Geometry check sheet. Reference: the model listing, model coordinates, mm. Round coordinates to 2 decimals unless told otherwise and drop trailing zeros. Order: outer loops, then holes, each group sorted by start corner. A loop starts at its lowest first (then second) coordinate and runs counter-clockwise, first axis right, second up. Notation, with made-up numbers: (60, 7.5) - (75, 7.5) arc R13 cw to (75, 23.5) - close; hole circle Ø5 at (-2.75, 37.25). An arc over 180 degrees is marked (long way). Return JSON: item names as keys, results as strings. Group by question number.
Q1. Material ranges on line 1 along Z through (x, y) = (-6, 3); line 2 along Y through (x, z) = (0, 8.75) (3 decimals); line 3 along X through (y, z) = (1, 5), recorded low to high.
Q2. Sectioned sample at A-A, the plane x = 0. Record the cut outline in (y, z) (3 decimals), then the cut area to 3 significant figures.
Q3. Gauge pin test, flat ends, axial feed: pin 1 Ø6 at (x, z) = (-8.5, 1) entering from +Y; pin 2 Ø5 at (x, z) = (-9.5, 4.5) entering from +Y; pin 3 Ø5 at (x, y) = (0, 0) entering from -Z; pin 4 Ø2 at (y, z) = (1, 2) entering from +X. Record the tip position at first contact, or that the pin passes through.
Q4. Draft check along Y on faces 1 (the cylindrical face through (-11.34, -0.65, 6.15)), 2 (the flat face through (-9.713, -0.012, -0.176)), 3 (the conical face through (9.553, 3.008, 5.127)), 4 (the cylindrical face through (-3.15, -2.41, 6.57)). Enter one of: pulls with the +Y half, pulls with the -Y half, needs draft (parallel to the pull), parting line crosses it, or undercut.
```python
from build123d import *

# Parameters (mm, degrees)
F0_R     = 8.895
F2_R     = 11.725
F4_R     = 3.965
F5_DEPTH = 12.95
F9_DEPTH = 13.225


with BuildPart() as f3:
    # F0 (on Top) → F3 section 0
    with BuildSketch(Plane.XY):
        Circle(F0_R)
    # F2 (on offset) → F3 section 1
    with BuildSketch(Plane.XY.offset(12.95)):
        Circle(F2_R)
    loft()

    # F4 (on face) → F5 (cut)
    with BuildSketch(Plane.XY.offset(12.95)):
        Circle(F4_R)
    extrude(amount=-F5_DEPTH, mode=Mode.SUBTRACT)

    # F8 (on face) → F9 (join)
    with BuildSketch(Plane(origin=(-0.370918, 0, 1.775485), x_dir=(0.978867, 0, 0.204496), z_dir=(0.204496, 0, -0.978867))):
        with BuildLine():
            ThreePointArc((-8.665283, 0.869945), (-9.857422, 0.644661), (-10.88518, -5.5e-05))
            ThreePointArc((-10.88518, -5.5e-05), (-9.857417, -0.644773), (-8.665273, -0.870055))
            ThreePointArc((-8.665273, -0.870055), (-8.707081, -5.6e-05), (-8.665283, 0.869945))
        make_face()
    extrude(amount=-F9_DEPTH)


solid = f3.part
```
Reply:
{
 "1": {"line 1": "0 to 12.95", "line 2": "-10.807 to -3.965, 3.965 to 10.807", "line 3": "-9.94 to -3.84, 3.84 to 9.94"},
 "2": {"outline": "(-11.725, 12.95) - (-8.895, 0) - (-3.965, 0) - (-3.965, 12.95) - close; (3.965, 0) - (8.895, 0) - (11.725, 12.95) - (3.965, 12.95) - close", "area": "164 mm^2"},
 "3": {"pin 1": "y = 7.41", "pin 2": "y = 7.09", "pin 3": "through", "pin 4": "x = 9.51"},
 "4": {"face 1": "pulls with the -Y half", "face 2": "needs draft", "face 3": "parting line crosses it", "face 4": "undercut"}
}
